Read the model definition and answer for the solid it produces. Units are mm, in the model's axes. Give positions to 0.01 mm unless a question says otherwise; leave off trailing zeros. Loops run counter-clockwise (first coordinate to the right, second up) from the corner with the lowest first, then second, coordinate; pieces in that order, holes last. Notation, with made-up numbers: (38.25, 7.25) - (53.25, 7.25) arc R26 cw to (53.25, 21.25) - close; hole circle Ø2 at (-0.75, 53). An arc over 180 degrees is marked (long way). Use a Markdown table: item, result. Add a question column.
Item 1: For a pull along Z with two mould halves and no side action, classify faces 1 (the face through (7, 16, 0)), 2 (the face through (12.031, 10.997, 8.131)), 3 (the face through (7, 16, 16)), 4 (the face through (7, 0, 8)) as +Z half, -Z half, draft (parallel to the pull), parting line (faces both ways), or undercut.
Item 2: A cutting plane is placed at B-B (x = 10.75). Determine the outline of the cut face in (y, z).
Item 3: A cutting plane is placed at A-A (y = 13). Determine the outline of the cut face in (x, z).
Item 4: A cutting plane is placed at D-D (x = 9.25). Determine the outline of the cut face in (y, z), plus the area to 3 significant figures.
Item 5: A cutting plane is placed at C-C (z = 7). Determine the outline of the cut face in (x, y), plus the area to 3 significant figures.
Item 6: This flat-tipped pin is pushed along its axis until it touches: P1, Ø3.5, axis at y = 13, z = 7.5, coming from the +X side. Where does it stop, or does it pass through?
Item 7: Consider probe 1 along Z at (x, y) = (1.5, 13); probe 2 along Y at (x, z) = (11.75, 7.5); probe 3 along X at (y, z) = (13, 5.25). Determine where each line is inside the solid, lowest interval first. Write a range as [from, to].
from build123d import *

# Parameters (mm, degrees)
F0_W     = 15
F0_H     = 26
F1_DEPTH = 16
F3_D     = 4.2
F5_D     = 4.2


with BuildPart() as f1:
    # F0 (on Top) → F1 (new body)
    with BuildSketch(Plane.XY):
        with Locations((7.5, 13)):
            Rectangle(F0_W, F0_H)
    extrude(amount=F1_DEPTH)

    # F3 (through all)
    with Locations(Plane.XY.offset(16)):
        with Locations((7.5, 13)):
            Hole(F3_D / 2)

    # F5 (through all)
    with Locations(Plane.YZ.offset(15)):
        with Locations((13, 7.5)):
            Hole(F5_D / 2)


solid = f1.part
Geometry says:
| question | item | result |
|---|---|---|
| 1 | face 1 | -Z half |
| 1 | face 2 | undercut |
| 1 | face 3 | +Z half |
| 1 | face 4 | draft |
| 2 | outline | (0, 0) - (26, 0) - (26, 16) - (0, 16) - close; hole circle Ø4.2 at (13, 7.5) |
| 3 | outline | (0, 0) - (5.4, 0) - (5.4, 5.4) - (0, 5.4) - close; (0, 9.6) - (5.4, 9.6) - (5.4, 16) - (0, 16) - close; (9.6, 0) - (15, 0) - (15, 5.4) - (9.6, 5.4) - close; (9.6, 9.6) - (15, 9.6) - (15, 16) - (9.6, 16) - close |
| 4 | outline | (0, 0) - (11.84, 0) - (11.84, 5.75) arc R2.1 cw to (11.84, 9.25) - (11.84, 16) - (0, 16) - close; (14.16, 0) - (26, 0) - (26, 16) - (14.16, 16) - (14.16, 9.25) arc R2.1 cw to (14.16, 5.75) - close |
| 4 | area | 374 mm² |
| 5 | outline | (0, 0) - (15, 0) - (15, 10.96) - (8, 10.96) arc R2.1 cw to (7, 10.96) - (0, 10.96) - close; (0, 15.04) - (7, 15.04) arc R2.1 cw to (8, 15.04) - (15, 15.04) - (15, 26) - (0, 26) - close |
| 5 | area | 329 mm² |
| 6 | P1 | through |
| 7 | probe 1 | [0, 5.4], [9.6, 16] |
| 7 | probe 2 | [0, 10.9], [15.1, 26] |
| 7 | probe 3 | [0, 5.4], [9.6, 15] |
